Source: CAD feature listing. Evaluate the final solid. Frame: model axes, mm. Face numbers are marked on the shaded views. Give positions to 0.01 mm unless a question says otherwise; leave off trailing zeros. Write each loop counter-clockwise with the first axis right and the second up, starting at its lowest first coordinate (ties: lowest second). Pieces come first, ordered by that corner, then holes. Notation, with made-up numbers: (66.25, 53.5) -> (115.25, 53.5) arc R33 ccw to (115.25, 87.5) -> close; hole circle Ø4 at (77, 64). An arc over 180 degrees is marked (long way). Write item = value, one per line.
from build123d import *

# Parameters (mm, degrees)
EXTRUDE_START         = -5
EXTRUDE_1_OUTLINE_R   = 1.5
EXTRUDE_1_DEPTH       = 5
EXTRUDE_1_2_OUTLINE_R = 1.5
EXTRUDE_1_2_DEPTH     = 5
SKETCH_2_R            = 14.5
SKETCH_2_R_2          = 12.5
EXTRUDE_2_DEPTH       = 13
SKETCH_3_R            = 14.5
SKETCH_3_R_2          = 12.5
EXTRUDE_5_DEPTH       = 2
SKETCH_4_W            = 16.5
SKETCH_4_H            = 160
SKETCH_4_W_2          = 12.5
SKETCH_4_H_2          = 156
EXTRUDE_4_DEPTH       = 12
CUT_EXTRUDE_1_REACH   = 265.836
EXTRUDE_6_DEPTH       = 60
EXTRUDE_7_DEPTH       = 60
SKETCH_12_W           = 16.582102221
SKETCH_12_H           = 6.424530869
SKETCH_12_W_2         = 10.745747925
SKETCH_12_H_2         = 9.027697981
CUT_EXTRUDE_2_DEPTH   = 60
SKETCH_14_W           = 16.5
SKETCH_14_H           = 160
SKETCH_14_W_2         = 12.5
SKETCH_14_H_2         = 156
EXTRUDE_8_DEPTH       = 2
SKETCH_16_R           = 3
SKETCH_16_R_2         = 1.5
EXTRUDE_9_DEPTH       = 5
CUT_EXTRUDE_START     = -5
SKETCH_17_R           = 1.5
CUT_EXTRUDE_3_DEPTH   = 5
SKETCH_18_R           = 1.5
CUT_EXTRUDE_4_DEPTH   = 5


with BuildPart() as part:
    # Extrude 1: read off the stored shape, not the designer's step
    # Extrude 1 outline → Extrude 1 (new body)
    with BuildSketch(Plane(origin=(0, 10.156954032, 0), x_dir=(1, 0, 0), z_dir=(0, 1, 0)).offset(EXTRUDE_START)):
        with BuildLine():
            Line((-54.445663034, -194.741719927), (-47.541721945, -196.591625367))
            ThreePointArc((-47.541721945, -196.591625367), (-43.67801864, -195.556349186), (-42.64274246, -191.692645881))
            Line((-42.64274246, -191.692645881), (-44.492647899, -184.788704792))
            ThreePointArc((-44.492647899, -184.788704792), (-44.796491977, -183.058763578), (-44.792972571, -181.302345222))
            ThreePointArc((-44.792972571, -181.302345222), (-48.981319499, -190.253048327), (-57.932022604, -194.441395255))
            ThreePointArc((-57.932022604, -194.441395255), (-56.175604248, -194.43787585), (-54.445663034, -194.741719927))
        make_face()
        with Locations((-46.506445765, -192.727922061)):
            Circle(EXTRUDE_1_OUTLINE_R, mode=Mode.SUBTRACT)
    extrude(amount=EXTRUDE_1_DEPTH)



with BuildPart() as body_2:
    # Extrude 1 2 outline → Extrude 1 2 (new body)
    with BuildSketch(Plane(origin=(0, 10.156954032, 0), x_dir=(1, 0, 0), z_dir=(0, 1, 0)).offset(EXTRUDE_START)):
        with BuildLine():
            Line((-64.023072619, -165.258280073), (-70.927013707, -163.408374633))
            ThreePointArc((-70.927013707, -163.408374633), (-74.790717013, -164.443650813), (-75.825993193, -168.307354119))
            Line((-75.825993193, -168.307354119), (-73.976087754, -175.211295208))
            ThreePointArc((-73.976087754, -175.211295208), (-73.672243676, -176.941236422), (-73.675763082, -178.697654778))
            ThreePointArc((-73.675763082, -178.697654778), (-69.487416154, -169.746951673), (-60.536713049, -165.558604745))
            ThreePointArc((-60.536713049, -165.558604745), (-62.293131405, -165.56212415), (-64.023072619, -165.258280073))
        make_face()
        with Locations((-71.962289888, -167.272077939)):
            Circle(EXTRUDE_1_2_OUTLINE_R, mode=Mode.SUBTRACT)
    extrude(amount=EXTRUDE_1_2_DEPTH)


with BuildPart() as part_1:
    add(part.part)

    add(body_2.part)  # Extrude 2 merges body 2
    # Sketch 2 → Extrude 2 (add)
    with BuildSketch(Plane.XZ.offset(-5.156954032)):
        with Locations(Location((-59.234367826, 180, 0), (0, 0, 270))):
            Circle(SKETCH_2_R)
        with Locations(Location((-59.234367826, 180, 0), (0, 0, 270))):
            Circle(SKETCH_2_R_2, mode=Mode.SUBTRACT)
    extrude(amount=-EXTRUDE_2_DEPTH)

    # Sketch 3 → Extrude 5 (add)
    # profile 1 of 4: a face of its own
    with BuildSketch(Plane(origin=(0, 18.156954032, 0), x_dir=(1, 0, 0), z_dir=(0, 1, 0))):
        with Locations(Location((-59.234367826, -180, 0), (0, 0, 95.153074257))):
            Circle(SKETCH_3_R)
        with Locations(Location((-59.234367826, -180, 0), (0, 0, 90))):
            Circle(SKETCH_3_R_2, mode=Mode.SUBTRACT)
    # profile 2 of 4: a face of its own
    with BuildSketch(Plane(origin=(0, 18.156954032, 0), x_dir=(1, 0, 0), z_dir=(0, 1, 0))):
        with BuildLine():
            Line((-73.734367826, -180), (-73.734367826, -260))
            Line((-73.734367826, -260), (-57.234367826, -260))
            Line((-57.234367826, -260), (-57.234367826, -194.361406616))
            ThreePointArc((-57.234367826, -194.361406616), (-68.754084209, -190.937321427), (-73.734367826, -180))
        make_face()
    # profile 3 of 4: a face of its own
    with BuildSketch(Plane(origin=(0, 18.156954032, 0), x_dir=(1, 0, 0), z_dir=(0, 1, 0))):
        with BuildLine():
            Line((-73.734367826, -100), (-73.734367826, -180))
            ThreePointArc((-73.734367826, -180), (-68.754084209, -169.062678573), (-57.234367826, -165.638593384))
            Line((-57.234367826, -165.638593384), (-57.234367826, -100))
            Line((-57.234367826, -100), (-73.734367826, -100))
        make_face()
    # profile 4 of 4: a face of its own
    with BuildSketch(Plane(origin=(0, 18.156954032, 0), x_dir=(1, 0, 0), z_dir=(0, 1, 0))):
        with BuildLine():
            Line((-59.234367826, -167.5), (-59.234367826, -192.5))
            ThreePointArc((-59.234367826, -192.5), (-50.395533062, -188.838834765), (-46.734367826, -180))
            ThreePointArc((-46.734367826, -180), (-50.395533062, -171.161165235), (-59.234367826, -167.5))
        make_face()
    extrude(amount=EXTRUDE_5_DEPTH)

    # Sketch 4 → Extrude 4 (add)
    with BuildSketch(Plane(origin=(0, 20.156954032, 0), x_dir=(1, 0, 0), z_dir=(0, 1, 0))):
        with Locations((-65.484367826, -180)):
            Rectangle(SKETCH_4_W, SKETCH_4_H)
        with Locations((-65.484367826, -180)):
            Rectangle(SKETCH_4_W_2, SKETCH_4_H_2, mode=Mode.SUBTRACT)
    extrude(amount=EXTRUDE_4_DEPTH)

    # Cut-Extrude 1: up to this face of the body (flat: up to its plane)
    cut_extrude_1_end = Plane(part_1.part.faces().sort_by_distance((-57.234367826, 26.156954032, 180))[0])
    # Sketch 7 → Cut-Extrude 1 (cut, up to the picked face)
    with BuildSketch(Plane.ZY.offset(73.734367826), mode=Mode.PRIVATE) as cut_extrude_1_sk1:
        Polygon((260, 30.156954032), (198.5, 18.156954032), (264.047822103, 13.706220506), (266.363809243, 29.164088167), align=None)
    cut_extrude_1_tool1 = split(extrude(cut_extrude_1_sk1.sketch, amount=-CUT_EXTRUDE_1_REACH, mode=Mode.PRIVATE), bisect_by=cut_extrude_1_end, keep=Keep.BOTH, mode=Mode.PRIVATE)
    # Sketch 7 → Cut-Extrude 1 (cut, up to the picked face)
    with BuildSketch(Plane.ZY.offset(73.734367826), mode=Mode.PRIVATE) as cut_extrude_1_sk2:
        Polygon((95.952177897, 13.706220506), (93.636190757, 29.164088167), (100, 30.156954032), (161.5, 18.156954032), align=None)
    cut_extrude_1_tool2 = split(extrude(cut_extrude_1_sk2.sketch, amount=-CUT_EXTRUDE_1_REACH, mode=Mode.PRIVATE), bisect_by=cut_extrude_1_end, keep=Keep.BOTH, mode=Mode.PRIVATE)
    add(cut_extrude_1_tool1.solids().sort_by(Axis((-73.734368, 20.991529, 242.810826), (1, 0, 0)))[0], mode=Mode.SUBTRACT)
    add(cut_extrude_1_tool2.solids().sort_by(Axis((-73.734368, 20.991529, 117.189174), (1, 0, 0)))[0], mode=Mode.SUBTRACT)



with BuildPart() as body_2_2:
    # Sketch 5 → Loft 1 section 0
    with BuildSketch(Plane(origin=(0, 32.156954032, 0), x_dir=(1, 0, 0), z_dir=(0, 1, 0))):
        with BuildLine():
            Line((-71.734367826, -258), (-59.234367826, -258))
            Line((-59.234367826, -258), (-59.234367826, -260))
            Line((-59.234367826, -260), (-71.734367826, -260))
            Line((-71.734367826, -260), (-71.734367826, -258))
        make_face()
    # Sketch 6 for Loft 1 → Loft 1 section 1
    with BuildSketch(Plane(origin=(0, 20.156954032, 0), x_dir=(1, 0, 0), z_dir=(0, 1, 0))):
        with BuildLine():
            Line((-71.734367826, -180), (-71.734367826, -190.770329614))
            # circular arc as an exact rational Bezier (weights 1, cos(half-angle), 1)
            Bezier((-71.734367826, -190.770329614), (-66.797532736, -196.5), (-59.234367826, -196.5), weights=[1, 0.909050947, 1])
            Line((-59.234367826, -196.5), (-59.234367826, -192.5))
            Bezier((-59.234367826, -192.5), (-71.734367826, -192.5), (-71.734367826, -180), weights=[1, 0.707106781, 1])
        make_face()
    loft()


with BuildPart() as part_2:
    add(part_1.part)

    add(body_2_2.part)  # Extrude 6 merges body 2 2
    # Sketch 8 → Extrude 6 (add, along a direction that is not the sketch's normal)
    with BuildSketch(Plane(origin=(0, 20.156954032, 0), x_dir=(1, 0, 0), z_dir=(0, 1, 0))):
        with BuildLine():
            Line((-71.734367826, -208.75), (-59.234367826, -208.75))
            Line((-59.234367826, -208.75), (-59.234367826, -192.5))
            ThreePointArc((-59.234367826, -192.5), (-68.073202591, -188.838834765), (-71.734367826, -180))
            Line((-71.734367826, -180), (-71.734367826, -208.75))
        make_face()
    extrude(amount=EXTRUDE_6_DEPTH, dir=(-6.810459085749413e-15, 0.1915103594196487, 0.9814905920256991))

    # Sketch 10 → Loft 2 section 0
    with BuildSketch(Plane(origin=(0, 32.156954032, 0), x_dir=(1, 0, 0), z_dir=(0, 1, 0))):
        with BuildLine():
            Line((-71.734367826, -102), (-59.234367826, -102))
            Line((-59.234367826, -102), (-59.234367826, -100))
            Line((-59.234367826, -100), (-71.734367826, -100))
            Line((-71.734367826, -100), (-71.734367826, -102))
        make_face()
    # Sketch 9 for Loft 2 → Loft 2 section 1
    with BuildSketch(Plane(origin=(0, 20.156954032, 0), x_dir=(1, 0, 0), z_dir=(0, 1, 0))):
        with BuildLine():
            Line((-71.734367826, -180), (-71.734367826, -169.229670386))
            Bezier((-71.734367826, -169.229670386), (-66.797532736, -163.5), (-59.234367826, -163.5), weights=[1, 0.909050947, 1])
            Line((-59.234367826, -163.5), (-59.234367826, -167.5))
            Bezier((-59.234367826, -167.5), (-71.734367826, -167.5), (-71.734367826, -180), weights=[1, 0.707106781, 1])
        make_face()
    loft()

    # Sketch 11 → Extrude 7 (add, along a direction that is not the sketch's normal)
    with BuildSketch(Plane(origin=(0, 20.156954032, 0), x_dir=(1, 0, 0), z_dir=(0, 1, 0))):
        with BuildLine():
            Line((-71.734367826, -151.25), (-71.734367826, -169.229670386))
            add(Edge.make_bspline(
                [(-71.734367826, -169.229670386), (-70.98639539, -168.36157667), (-70.129603224, -167.552057992), (-68.236734624, -166.121426347), (-67.200962736, -165.500879161), (-65.018377367, -164.50043958), (-63.872168611, -164.120824376), (-61.552791986, -163.620673884), (-60.380251531, -163.5), (-59.234367826, -163.5)],
                knots=[0, 0, 0, 0, 0.25, 0.25, 0.5, 0.5, 0.75, 0.75, 1, 1, 1, 1], degree=3))
            Line((-59.234367826, -163.5), (-59.234367826, -151.25))
            Line((-59.234367826, -151.25), (-71.734367826, -151.25))
        make_face()
    extrude(amount=EXTRUDE_7_DEPTH, dir=(0, 0.1915103594196487, -0.9814905920256991))

    # Sketch 12 → Cut-Extrude 2 (cut)
    with BuildSketch(Plane(origin=(-57.234367826, 0, 0), x_dir=(0, 0, -1), z_dir=(1, 0, 0))):
        with Locations((-91.708948889, 28.944688598)):
            Rectangle(SKETCH_12_W, SKETCH_12_H)
        with Locations((-265.372873962, 27.643105042)):
            Rectangle(SKETCH_12_W_2, SKETCH_12_H_2)
    extrude(amount=-CUT_EXTRUDE_2_DEPTH, mode=Mode.SUBTRACT)

    # Sketch 14 → Extrude 8 (add)
    with BuildSketch(Plane(origin=(0, 32.156954032, 0), x_dir=(1, 0, 0), z_dir=(0, 1, 0))):
        with Locations((-65.484367826, -180)):
            Rectangle(SKETCH_14_W, SKETCH_14_H)
        with Locations((-65.484367826, -180)):
            Rectangle(SKETCH_14_W_2, SKETCH_14_H_2, mode=Mode.SUBTRACT)
    extrude(amount=EXTRUDE_8_DEPTH)

    # Sketch 16 → Extrude 9 (add)
    with BuildSketch(Plane(origin=(0, 47.847472623, 9.336092219), x_dir=(1, 0, 0), z_dir=(0, -0.981490592025699, -0.19151035941964872))):
        with Locations(Location((-65.484367826, 102.572898444, 0), (0, 0, 90))):
            Circle(SKETCH_16_R)
        with Locations(Location((-65.484367826, 102.572898444, 0), (0, 0, 270))):
            Circle(SKETCH_16_R_2, mode=Mode.SUBTRACT)
    extrude_9 = extrude(amount=EXTRUDE_9_DEPTH)

    # Sketch 17 → Cut-Extrude 3 (cut)
    with BuildSketch(Plane(origin=(0, 47.847472623, 9.336092219), x_dir=(1, 0, 0), z_dir=(0, -0.981490592025699, -0.19151035941964872)).offset(CUT_EXTRUDE_START)):
        with Locations(Location((-65.484367826, 102.572898444, 0), (0, 0, 57.025282915))):
            Circle(SKETCH_17_R)
    extrude(amount=CUT_EXTRUDE_3_DEPTH, mode=Mode.SUBTRACT)

    # Mirror 1: Extrude 9 across plane
    add(extrude_9.mirror(Plane(origin=(0, 0, 180), x_dir=(1, 0, 0), z_dir=(0, 0, -1))))

    # Sketch 18 → Cut-Extrude 4 (cut)
    with BuildSketch(Plane(origin=(0, -19.820149153, 3.867346176), x_dir=(1, 0, 0), z_dir=(-4.422479578024356e-14, -0.981490592025698, 0.1915103594196541)).offset(CUT_EXTRUDE_START)):
        with Locations(Location((-65.484367826, 250.763714686, 0), (0, 0, 90))):
            Circle(SKETCH_18_R)
    extrude(amount=CUT_EXTRUDE_4_DEPTH, mode=Mode.SUBTRACT)


solid = part_2.part
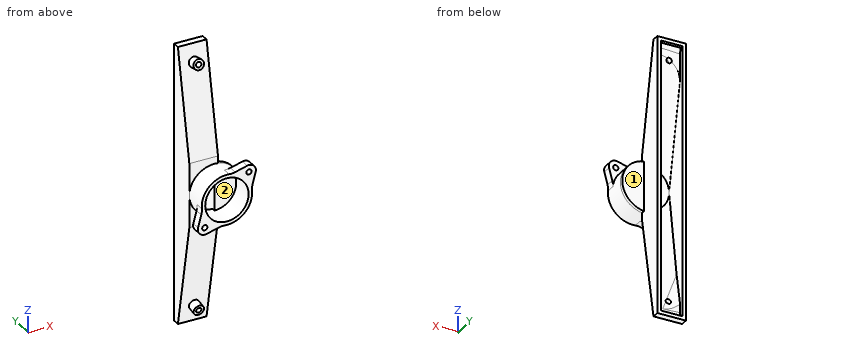
(1) Material intervals for line 1 (X direction, y = 30, z = 230.5); line 2 (X direction, y = 11.5, z = 180); line 3 (Z direction, x = -60, y = 8.25), sorted ascending.
Values follow:
line_1 = -73.73 to -71.73, -59.23 to -57.23
line_2 = -73.73 to -71.73, -46.73 to -44.73
line_3 = 165.52 to 167.52, 192.48 to 194.48
(2) First-contact query: pin 1 (8 mm diameter, centred on y = 25, z = 215.5, fed in from -X); pin 2 (0.8 mm diameter, centred on x = -67.5, z = 102.5, fed in from +Y); pin 3 (10 mm diameter, centred on x = -68, z = 243, fed in from +Y); pin 4 (1.5 mm diameter, centred on y = 26, z = 218, fed in from +X). Flat tips, straight axial feed; report the tip coordinate or a pass-through.
Values follow:
pin_1 = -73.73
pin_2 = 32.14
pin_3 = 34.16
pin_4 = -57.23
(3) Section query B-B (x = -53). Return loops of the section in (y, z).
Values follow:
outline = (5.16, 166.91) -> (20.16, 166.91) -> (20.16, 193.09) -> (10.16, 193.09) -> (10.16, 195.13) -> (5.16, 195.13) -> (5.16, 190.83) -> (18.16, 190.83) -> (18.16, 169.17) -> (5.16, 169.17) -> close
(4) Pull-direction query (Z, two-part tool) for the marked faces 1 and 2; classes: pulls with the +Z half, pulls with the -Z half, needs draft (parallel to the pull), parting line crosses it, or undercut.
Values follow:
face_1 = needs draft
face_2 = undercut
(5) Section query A-A (y = 15.5). Return loops of the section in (x, z).
Values follow:
outline = circle Ø29 at (-59.23, 180); hole circle Ø25 at (-59.23, 180)
